from build123d import *

# Parameters (mm, degrees)
BOSS_EXTRUDE1_DEPTH     = 1.6002
F_1_4_CLEARANCE_HOLE1_D = 7.14248


with BuildPart() as part:
    # Sketch1 → Boss-Extrude1 (new body)
    with BuildSketch(Plane.XY):
        Polygon((63.5, 76.2), (133.35, 76.2), (133.35, -76.2), (-133.35, -76.2), (-133.35, 76.2), (-63.5, 76.2), (-63.5, 0), (63.5, 0), align=None)
    extrude(amount=BOSS_EXTRUDE1_DEPTH)

    # 1/4 Clearance Hole1 (through all)
    with Locations(Plane.XY.offset(1.6002)):
        with Locations((-107.95, 31.75), (107.95, 31.75)):
            Hole(F_1_4_CLEARANCE_HOLE1_D / 2)


solid = part.part
Check sheet for the modelled part. Datum: model origin and axes. Units: mm. Round coordinates to 2 decimals unless told otherwise and drop trailing zeros. Loops run counter-clockwise (first coordinate to the right, second up) from the corner with the lowest first, then second, coordinate; pieces in that order, holes last.
1. Sectioned sample at A-A on y = 31.75. Record the boundary of the cut face in (x, z).
2. Scan lines: probe 1 along X at (y, z) = (46.5, 1.3); probe 2 along Y at (x, z) = (-107.95, 1.3); probe 3 along Y at (x, z) = (-36.5, 0.4). Record each from-to range of solid material in increasing order.
3. Sectioned sample at B-B on z = 1.25. Record the boundary of the cut face in (x, y).
4. Gauge pin test, flat end, axial feed: pin 1 Ø0.8 at (x, z) = (22, 0.5) entering from +Y. Record the tip position at first contact, or that the pin passes through.
5. Mould release check, pull along Y, two halves, no side actions. Record for faces 1 (the cylindrical face through (-104.382, 31.907, 0.789)), 2 (the cylindrical face through (106.03, 34.76, 0.79)), 3 (the flat face through (2, -16, 1.6)): released by +Y, released by -Y, zero draft, split by the parting line, or undercut.
6. Sectioned sample at C-C on x = 107.95. Record the boundary of the cut face in (y, z), and give its area (3 significant figures).
7. Sectioned sample at D-D on x = -25.5. Record the boundary of the cut face in (y, z).
Recorded:
1. outline: (-133.35, 0) - (-111.52, 0) - (-111.52, 1.6) - (-133.35, 1.6) - close; (-104.38, 0) - (-63.5, 0) - (-63.5, 1.6) - (-104.38, 1.6) - close; (63.5, 0) - (104.38, 0) - (104.38, 1.6) - (63.5, 1.6) - close; (111.52, 0) - (133.35, 0) - (133.35, 1.6) - (111.52, 1.6) - close
2. probe 1: x = -133.35 to -63.5, 63.5 to 133.35
2. probe 2: y = -76.2 to 28.18, 35.32 to 76.2
2. probe 3: y = -76.2 to 0
3. outline: (-133.35, -76.2) - (133.35, -76.2) - (133.35, 76.2) - (63.5, 76.2) - (63.5, 0) - (-63.5, 0) - (-63.5, 76.2) - (-133.35, 76.2) - close; hole circle Ø7.14 at (-107.95, 31.75); hole circle Ø7.14 at (107.95, 31.75)
4. pin 1: stops at y = 0
5. face 1: undercut
5. face 2: undercut
5. face 3: zero draft
6. outline: (-76.2, 0) - (28.18, 0) - (28.18, 1.6) - (-76.2, 1.6) - close; (35.32, 0) - (76.2, 0) - (76.2, 1.6) - (35.32, 1.6) - close
6. area: 232 mm2
7. outline: (-76.2, 0) - (0, 0) - (0, 1.6) - (-76.2, 1.6) - close
